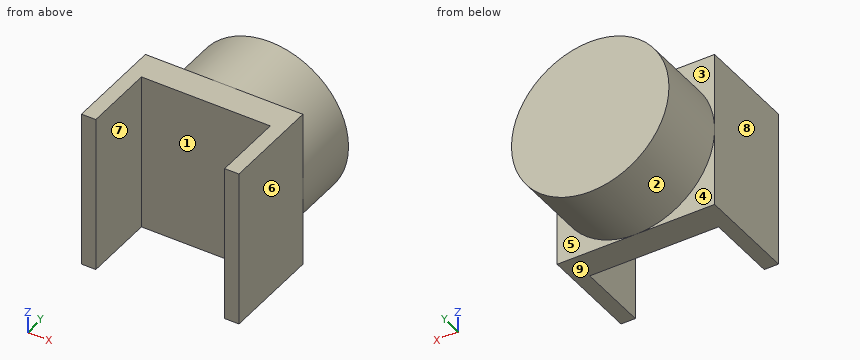
```python
from build123d import *

# Parameters (mm, degrees)
SKETCH1_R           = 5.5
BOSS_EXTRUDE1_DEPTH = 5
SKETCH2_W           = 11
SKETCH2_H           = 11
BOSS_EXTRUDE2_DEPTH = 2
SKETCH3_W           = 1
SKETCH3_H           = 11
BOSS_EXTRUDE3_DEPTH = 5


with BuildPart() as part:
    # Sketch1 → Boss-Extrude1 (new body)
    with BuildSketch(Plane(origin=(0, 0, 0), x_dir=(1, 0, 0), z_dir=(0, 1, 0))):
        with Locations(Location((0, 0, 0), (0, 0, 270))):
            Circle(SKETCH1_R)
    extrude(amount=BOSS_EXTRUDE1_DEPTH)

    # Sketch2 → Boss-Extrude2 (add)
    with BuildSketch(Plane(origin=(0, 0, 0), x_dir=(-1, 0, 0), z_dir=(0, -1, 0))):
        Rectangle(SKETCH2_W, SKETCH2_H)
    extrude(amount=BOSS_EXTRUDE2_DEPTH)

    # Sketch3 → Boss-Extrude3 (add)
    with BuildSketch(Plane(origin=(0, -2, 0), x_dir=(-1, 0, 0), z_dir=(0, -1, 0))):
        with Locations((5, 0)):
            Rectangle(SKETCH3_W, SKETCH3_H)
        with Locations((-5, 0)):
            Rectangle(SKETCH3_W, SKETCH3_H)
    extrude(amount=BOSS_EXTRUDE3_DEPTH)


solid = part.part
```
Check sheet for the modelled part. Datum: model origin and axes. Units: mm. Face numbers are marked on the shaded views. A direction names the side the tool comes from. Give positions to 0.01 mm unless a question says otherwise; leave off trailing zeros. Loops run counter-clockwise (first coordinate to the right, second up) from the corner with the lowest first, then second, coordinate; pieces in that order, holes last. Notation, with made-up numbers: M 30.5,-14 L 46.5,-14 A37 ccw 46.5,24 Z; hole C -34,68.5 d5. An arc over 180 degrees is marked long. Answer in a Markdown table with one row per item.
1) Thickness scan on line 1 (X direction, y = -4, z = 2.5); line 2 (Y direction, x = 5, z = 3); line 3 (Y direction, x = 2.25, z = 3.5). Record the ranges inside material, lowest first.
Solutions:
| item | result |
|---|---|
| line 1 | x = -5.5 to -4.5, 4.5 to 5.5 |
| line 2 | y = -7 to 0 |
| line 3 | y = -2 to 5 |
2) Cross-section at B-B (z = 3). Enter the section's corners in (x, y), plus the area to 3 significant figures.
Solutions:
| item | result |
|---|---|
| outline | M -5.5,-7 L -4.5,-7 L -4.5,-2 L 4.5,-2 L 4.5,-7 L 5.5,-7 L 5.5,0 L 4.61,0 L 4.61,5 L -4.61,5 L -4.61,0 L -5.5,0 Z |
| area | 78.1 mm^2 |
3) Tool access check on the marked faces 1, 2, 3, 4 and 5. Record the directions out of +Z, -Z, +X, -X, +Y, -Y that give a thin tool (end or side, any length) a straight path to the whole face; none if there is none.
Solutions:
| item | result |
|---|---|
| face 1 | +Z, -Z, -Y |
| face 2 | +Y |
| face 3 | +Z, -X, +Y |
| face 4 | -Z, -X, +Y |
| face 5 | -Z, +X, +Y |
4) Mould release check, pull along X, two halves, no side actions. Record for the marked faces 6, 7, 8 and 9: released by +X, released by -X, zero draft, split by the parting line, or undercut.
Solutions:
| item | result |
|---|---|
| face 6 | released by +X |
| face 7 | undercut |
| face 8 | released by -X |
| face 9 | zero draft |
5) Cross-section at D-D (x = -3). Enter the section's corners in (y, z), plus the area to 3 significant figures.
Solutions:
| item | result |
|---|---|
| outline | M -2,-5.5 L 0,-5.5 L 0,-4.61 L 5,-4.61 L 5,4.61 L 0,4.61 L 0,5.5 L -2,5.5 Z |
| area | 68.1 mm^2 |
6) Cross-section at A-A (y = -4.25). Enter the section's corners in (x, z).
Solutions:
| item | result |
|---|---|
| outline | M -5.5,-5.5 L -4.5,-5.5 L -4.5,5.5 L -5.5,5.5 Z; M 4.5,-5.5 L 5.5,-5.5 L 5.5,5.5 L 4.5,5.5 Z |
